from build123d import *

# Parameters (mm, degrees)
BOSS_EXTRUDE1_DEPTH      = 2
BOSS_EXTRUDE1_DEPTH_BACK = 5
SKETCH1_W                = 20
SKETCH1_H                = 24.4
CUT_EXTRUDE1_DEPTH       = 24.954957733
SKETCH4_R                = 4.5
BOSS_EXTRUDE2_DEPTH      = 1.2
SKETCH5_R                = 2.6
BOSS_EXTRUDE3_DEPTH      = 6


with BuildPart() as part:
    # Sketch1 → Boss-Extrude1 (new, two sides: drawn at the far end of the back side and taken through both)
    with BuildSketch(Plane.XY.offset(-BOSS_EXTRUDE1_DEPTH_BACK)):
        Rectangle(SKETCH1_W, SKETCH1_H)
    extrude(amount=BOSS_EXTRUDE1_DEPTH + BOSS_EXTRUDE1_DEPTH_BACK)

    # Sketch3 → Cut-Extrude1 (cut, through all)
    with BuildSketch(Plane(origin=(10, 0, 0), x_dir=(0, 0, -1), z_dir=(1, 0, 0))):
        Polygon((8.2, -10.4), (1.439444872, -10.4), (-0.2, -9.307036752), (-0.2, -7.95), (-0.2, -5.45), (-0.2, 5.45), (-0.2, 7.95), (-0.2, 9.307036752), (1.439444872, 10.4), (8.2, 10.4), align=None)
    extrude(amount=-CUT_EXTRUDE1_DEPTH, mode=Mode.SUBTRACT)

    # Sketch4 → Boss-Extrude2 (add)
    with BuildSketch(Plane.XY.offset(2)):
        Circle(SKETCH4_R)
    extrude(amount=BOSS_EXTRUDE2_DEPTH)

    # Sketch5 → Boss-Extrude3 (add)
    with BuildSketch(Plane.XY.offset(3.2)):
        Circle(SKETCH5_R)
    extrude(amount=BOSS_EXTRUDE3_DEPTH)


solid = part.part
Here's how the part is built. I have some questions about the finished solid (model axes, mm). A direction names the side the tool comes from. Coordinates: 2 decimals unless noted, no trailing zeros. Write each loop counter-clockwise with the first axis right and the second up, starting at its lowest first coordinate (ties: lowest second). Pieces come first, ordered by that corner, then holes.
1) If I drill on line 1 (Y direction, x = -6.5, z = -3); line 2 (Z direction, x = -8.25, y = 4.75); line 3 (Z direction, x = -2.5, y = 2), over which ranges is the centre line in solid material (lowest first)?
Filled in:
line 1: y = -12.2 to -10.4, 10.4 to 12.2
line 2: z = 0.2 to 2
line 3: z = 0.2 to 3.2
2) If we section it at D-D (z = 4.75): List the corners of the cut face in (x, y) for me, plus the area to 3 significant figures.
Filled in:
outline: circle Ø5.2 at (0, 0)
area: 21.2 mm2
3) If we section it at B-B (y = 0): List the corners of the cut face in (x, z) for me.
Filled in:
outline: (-10, 0.2) - (10, 0.2) - (10, 2) - (4.5, 2) - (4.5, 3.2) - (2.6, 3.2) - (2.6, 9.2) - (-2.6, 9.2) - (-2.6, 3.2) - (-4.5, 3.2) - (-4.5, 2) - (-10, 2) - close
4) Which directions (+Z, -Z, +X, -X, +Y, -Y) give clear straight access to the entire face, cutting with the end or side of a thin tool? Please do faces 4 (the face through (0, 11, -5)), 5 (the face through (0, 10.4, -3)), 6 (the face through (-0.338, 2.578, 6.158)).
Filled in:
face 4: -Z, +X, -X, +Y, -Y
face 5: -Z, +X, -X
face 6: +Z
5) If we section it at C-C (x = 0): List the corners of the cut face in (y, z) for me, plus the area to 3 significant figures.
Filled in:
outline: (-12.2, -5) - (-10.4, -5) - (-10.4, -1.44) - (-9.31, 0.2) - (9.31, 0.2) - (10.4, -1.44) - (10.4, -5) - (12.2, -5) - (12.2, 2) - (4.5, 2) - (4.5, 3.2) - (2.6, 3.2) - (2.6, 9.2) - (-2.6, 9.2) - (-2.6, 3.2) - (-4.5, 3.2) - (-4.5, 2) - (-12.2, 2) - close
area: 106 mm2
6) If we section it at A-A (z = -3.25): List the corners of the cut face in (x, y) for me.
Filled in:
outline: (-10, -12.2) - (10, -12.2) - (10, -10.4) - (-10, -10.4) - close; (-10, 10.4) - (10, 10.4) - (10, 12.2) - (-10, 12.2) - close
7) I'm going to push flat-ended pins straight in: pin 1 (1.5 mm diameter, centred on x = 5.5, y = 0, fed in from +Z); pin 2 (4 mm diameter, centred on x = -3, z = 6, fed in from -Y); pin 3 (5 mm diameter, centred on x = -3, y = -0.5, fed in from -Z). Where does each tip first touch, or does it pass through?
Filled in:
pin 1: stops at z = 2
pin 2: stops at y = -2.4
pin 3: stops at z = 0.2
8) Thinking about a two-plate mould opening in Y: for faces 1 (the face through (0, 0, 0.2)), 2 (the face through (0, 0, 9.2)), 3 (the face through (-0.59, 4.46, 2.59)), which applies, +Y half, -Y half, draft (parallel to the pull), parting line (faces both ways), or undercut?
Filled in:
face 1: undercut
face 2: draft
face 3: parting line
